from build123d import *

# Parameters (mm, degrees)
SKETCH1_R           = 92.5
BOSS_EXTRUDE1_DEPTH = 5
BOSS_EXTRUDE2_DEPTH = 5
CUT_EXTRUDE4_REACH  = 12
SKETCH13_R          = 2.25


with BuildPart() as part:
    # Sketch1 → Boss-Extrude1 (new body)
    with BuildSketch(Plane.XY):
        Circle(SKETCH1_R)
    extrude(amount=BOSS_EXTRUDE1_DEPTH)

    # Sketch12 → Boss-Extrude2 (add)
    with BuildSketch(Plane.XY.offset(5)):
        Polygon((62.861769108, -20.84153395), (67.861769108, -20.84153395), (67.861769108, 46.15846605), (62.861769108, 46.15846605), (62.861769108, 51.15846605), (72.861769108, 51.15846605), (72.861769108, -25.84153395), (62.861769108, -25.84153395), align=None)
        Polygon((11.861769105, 46.15846605), (11.861769105, -20.84153395), (16.861769105, -20.84153395), (16.861769105, -25.84153395), (6.861769105, -25.84153395), (6.861769105, 51.15846605), (16.861769105, 51.15846605), (16.861769105, 46.15846605), align=None)
    extrude(amount=BOSS_EXTRUDE2_DEPTH)

    # Sketch13 → Cut-Extrude4 (cut, up to next)
    with BuildSketch(Plane(origin=(0, 0, 0), x_dir=(-1, 0, 0), z_dir=(0, 0, -1)), mode=Mode.PRIVATE) as cut_extrude4_sk1:
        with Locations((-87.5, 0)):
            Circle(SKETCH13_R)
    cut_extrude4_tool1 = extrude(cut_extrude4_sk1.sketch, amount=-CUT_EXTRUDE4_REACH, mode=Mode.PRIVATE) & part.part
    add(cut_extrude4_tool1.solids().sort_by_distance((87.5, 0, 0))[0], mode=Mode.SUBTRACT)
    # Sketch13 → Cut-Extrude4 (cut, up to next)
    with BuildSketch(Plane(origin=(0, 0, 0), x_dir=(-1, 0, 0), z_dir=(0, 0, -1)), mode=Mode.PRIVATE) as cut_extrude4_sk2:
        with Locations((-61.871843354, 61.871843354)):
            Circle(SKETCH13_R)
    cut_extrude4_tool2 = extrude(cut_extrude4_sk2.sketch, amount=-CUT_EXTRUDE4_REACH, mode=Mode.PRIVATE) & part.part
    add(cut_extrude4_tool2.solids().sort_by_distance((61.871843, 61.871843, 0))[0], mode=Mode.SUBTRACT)
    # Sketch13 → Cut-Extrude4 (cut, up to next)
    with BuildSketch(Plane(origin=(0, 0, 0), x_dir=(-1, 0, 0), z_dir=(0, 0, -1)), mode=Mode.PRIVATE) as cut_extrude4_sk3:
        with Locations((0, 87.5)):
            Circle(SKETCH13_R)
    cut_extrude4_tool3 = extrude(cut_extrude4_sk3.sketch, amount=-CUT_EXTRUDE4_REACH, mode=Mode.PRIVATE) & part.part
    add(cut_extrude4_tool3.solids().sort_by_distance((0, 87.5, 0))[0], mode=Mode.SUBTRACT)
    # Sketch13 → Cut-Extrude4 (cut, up to next)
    with BuildSketch(Plane(origin=(0, 0, 0), x_dir=(-1, 0, 0), z_dir=(0, 0, -1)), mode=Mode.PRIVATE) as cut_extrude4_sk4:
        with Locations((61.871843354, 61.871843354)):
            Circle(SKETCH13_R)
    cut_extrude4_tool4 = extrude(cut_extrude4_sk4.sketch, amount=-CUT_EXTRUDE4_REACH, mode=Mode.PRIVATE) & part.part
    add(cut_extrude4_tool4.solids().sort_by_distance((-61.871843, 61.871843, 0))[0], mode=Mode.SUBTRACT)
    # Sketch13 → Cut-Extrude4 (cut, up to next)
    with BuildSketch(Plane(origin=(0, 0, 0), x_dir=(-1, 0, 0), z_dir=(0, 0, -1)), mode=Mode.PRIVATE) as cut_extrude4_sk5:
        with Locations((87.5, 0)):
            Circle(SKETCH13_R)
    cut_extrude4_tool5 = extrude(cut_extrude4_sk5.sketch, amount=-CUT_EXTRUDE4_REACH, mode=Mode.PRIVATE) & part.part
    add(cut_extrude4_tool5.solids().sort_by_distance((-87.5, 0, 0))[0], mode=Mode.SUBTRACT)
    # Sketch13 → Cut-Extrude4 (cut, up to next)
    with BuildSketch(Plane(origin=(0, 0, 0), x_dir=(-1, 0, 0), z_dir=(0, 0, -1)), mode=Mode.PRIVATE) as cut_extrude4_sk6:
        with Locations((61.871843354, -61.871843354)):
            Circle(SKETCH13_R)
    cut_extrude4_tool6 = extrude(cut_extrude4_sk6.sketch, amount=-CUT_EXTRUDE4_REACH, mode=Mode.PRIVATE) & part.part
    add(cut_extrude4_tool6.solids().sort_by_distance((-61.871843, -61.871843, 0))[0], mode=Mode.SUBTRACT)
    # Sketch13 → Cut-Extrude4 (cut, up to next)
    with BuildSketch(Plane(origin=(0, 0, 0), x_dir=(-1, 0, 0), z_dir=(0, 0, -1)), mode=Mode.PRIVATE) as cut_extrude4_sk7:
        with Locations((0, -87.5)):
            Circle(SKETCH13_R)
    cut_extrude4_tool7 = extrude(cut_extrude4_sk7.sketch, amount=-CUT_EXTRUDE4_REACH, mode=Mode.PRIVATE) & part.part
    add(cut_extrude4_tool7.solids().sort_by_distance((0, -87.5, 0))[0], mode=Mode.SUBTRACT)
    # Sketch13 → Cut-Extrude4 (cut, up to next)
    with BuildSketch(Plane(origin=(0, 0, 0), x_dir=(-1, 0, 0), z_dir=(0, 0, -1)), mode=Mode.PRIVATE) as cut_extrude4_sk8:
        with Locations((-61.871843354, -61.871843354)):
            Circle(SKETCH13_R)
    cut_extrude4_tool8 = extrude(cut_extrude4_sk8.sketch, amount=-CUT_EXTRUDE4_REACH, mode=Mode.PRIVATE) & part.part
    add(cut_extrude4_tool8.solids().sort_by_distance((61.871843, -61.871843, 0))[0], mode=Mode.SUBTRACT)


solid = part.part
Part model, mm, in its own coordinate system. A direction names the side the tool comes from. Give positions to 0.01 mm unless a question says otherwise; leave off trailing zeros. Write each loop counter-clockwise with the first axis right and the second up, starting at its lowest first coordinate (ties: lowest second). Pieces come first, ordered by that corner, then holes.
1) Two-plate mould, pull along Y, no slides. Class faces 6 (the face through (14, 46.158, 7)), 7 (the face through (49.727, 77.996, 2.465)), 8 (the face through (6.862, 12, 7)), 9 (the face through (85.42, -0.86, 2.46)): released by +Y, released by -Y, zero draft, split by the parting line, or undercut.
Resolved:
face 6: undercut
face 7: split by the parting line
face 8: zero draft
face 9: undercut
2) Pin check, flat tips, straight feed: pin 1 (7 mm diameter, centred on x = 87.5, y = 0, fed in from -Z); pin 2 (5.5 mm diameter, centred on x = 65.5, z = 7.5, fed in from -Y); pin 3 (1.5 mm diameter, centred on x = 67.5, z = 8.5, fed in from +Y); pin 4 (5.5 mm diameter, centred on y = 22, z = 8.5, fed in from +X). Stop position of each tip, or through.
Resolved:
pin 1: stops at z = 0
pin 2: stops at y = -66.44
pin 3: stops at y = 51.16
pin 4: stops at x = 72.86
3) Probe L1, parallel to Y at x = 0, z = 1.45; L2, parallel to Z at x = -34, y = -51; L3, parallel to Y at x = 67.5, z = 6. List the from-to ranges inside material, lowest first.
Resolved:
L1: y = -92.5 to -89.75, -85.25 to 85.25, 89.75 to 92.5
L2: z = 0 to 5
L3: y = -25.84 to -20.84, 46.16 to 51.16
4) Cut at A-A on y = 87.5. Write the cut outline in (x, z), then the cut area to 4 significant figures.
Resolved:
outline: (-30, 0) - (-2.25, 0) - (-2.25, 5) - (-30, 5) - close; (2.25, 0) - (30, 0) - (30, 5) - (2.25, 5) - close
area: 277.5 mm2
5) Cut at D-D on z = 6.5. Write the cut outline in (x, y), then the cut area to 3 significant figures.
Resolved:
outline: (6.86, -25.84) - (16.86, -25.84) - (16.86, -20.84) - (11.86, -20.84) - (11.86, 46.16) - (16.86, 46.16) - (16.86, 51.16) - (6.86, 51.16) - close; (62.86, -25.84) - (72.86, -25.84) - (72.86, 51.16) - (62.86, 51.16) - (62.86, 46.16) - (67.86, 46.16) - (67.86, -20.84) - (62.86, -20.84) - close
area: 870 mm2
6) Cut at B-B on x = 0. Write the cut outline in (y, z), then the cut area to 3 significant figures.
Resolved:
outline: (-92.5, 0) - (-89.75, 0) - (-89.75, 5) - (-92.5, 5) - close; (-85.25, 0) - (85.25, 0) - (85.25, 5) - (-85.25, 5) - close; (89.75, 0) - (92.5, 0) - (92.5, 5) - (89.75, 5) - close
area: 880 mm2
7) Which spindle directions (+Z, -Z, +X, -X, +Y, -Y) get a long thin tool onto all of the face, cutting with end or side? Do faces 1 (the face through (69, 13, 10)), 2 (the face through (68, 51.158, 7)), 3 (the face through (60.662, 63.769, 2.465)), 4 (the face through (14, -20.842, 7)), 5 (the face through (16.862, -23, 7)). Say none if no direction does.
Resolved:
face 1: +Z, +X, -X, +Y, -Y
face 2: +Z, +X, -X, +Y
face 3: +Z, -Z
face 4: +Z
face 5: +Z, +Y, -Y
